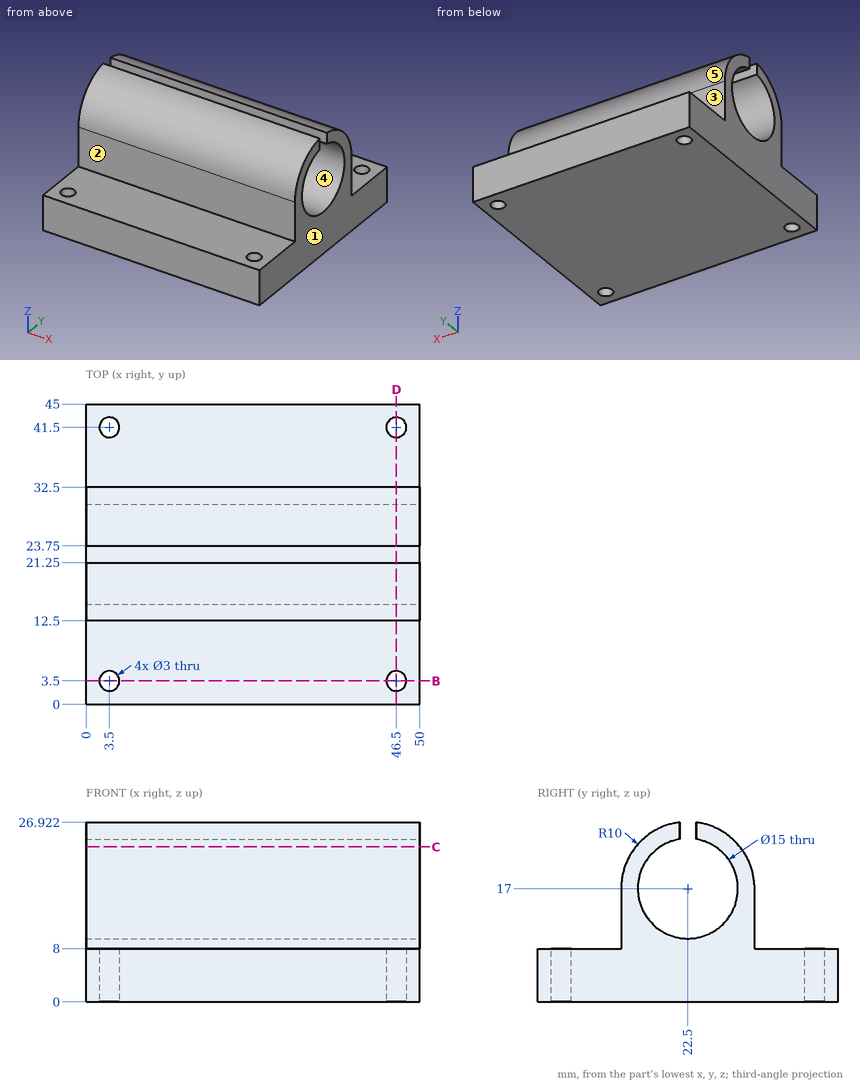
Can you work these out from the drawing? Everything is in mm from the part's minimum corner. A direction names the side the tool comes from. Round coordinates to 2 decimals unless told otherwise and drop trailing zeros. Write each loop counter-clockwise with the first axis right and the second up, starting at its lowest first coordinate (ties: lowest second). Pieces come first, ordered by that corner, then holes.
1. If we mould it in two halves opening along Z, with no side actions, what happens to the marked faces 3, 4 and 5? For each: released by +Z, released by -Z, zero draft, split by the parting line, or undercut.
2. For the marked faces 1 and 2, which set-ups out of +Z, -Z, +X, -X, +Y, -Y let a thin tool reach every point of the face, with its end or its side?
3. Will these pins go through, and if not, where does the flat tip stop? pin 1 Ø2.5 at (x, y) = (3.5, 3.5) entering from -Z; pin 2 Ø1.3 at (x, z) = (22, 25.5) entering from -Y (1 decimal); pin 3 Ø4 at (x, z) = (32, 13.5) entering from -Y; pin 4 Ø4 at (x, y) = (22.5, 7.5) entering from +Z.
4. Suppose I cut it at B-B (y = 3.5). List the corners of the cut face in (x, z) for me.
5. Suppose I cut it at D-D (x = 46.5). State how many separate pieces and enclosed holes the cut face has, and give its area (3 significant figures).
6. Suppose I cut it at C-C (z = 23.25). List the corners of the cut face in (x, y) for me (1 decimal), and give its area (3 significant figures).
7. I need wall thicknesses on L1, parallel to Y at x = 3.5, z = 3; L2, parallel to Y at x = 39, z = 17; L3, parallel to Y at x = 47, z = 1.75 (1 decimal). Which ranges of each line are inside material? Lowest first, please.
Answer sheet:
1. face 3: zero draft
1. face 4: undercut
1. face 5: released by +Z
2. face 1: +Z, -Z, +X, +Y, -Y
2. face 2: +Z, +X, -X, -Y
3. pin 1: passes through
3. pin 2: stops at y = 16.3
3. pin 3: stops at y = 12.5
3. pin 4: stops at z = 8
4. outline: (0, 0) - (2, 0) - (2, 8) - (0, 8) - close; (5, 0) - (45, 0) - (45, 8) - (5, 8) - close; (48, 0) - (50, 0) - (50, 8) - (48, 8) - close
5. separate pieces: 3
5. enclosed holes: 0
5. area: 466 mm2
6. outline: (0, 14.7) - (50, 14.7) - (50, 18.4) - (0, 18.4) - close; (0, 26.6) - (50, 26.6) - (50, 30.3) - (0, 30.3) - close
6. area: 366 mm2
7. L1: y = 0 to 2, 5 to 40, 43 to 45
7. L2: y = 12.5 to 15, 30 to 32.5
7. L3: y = 0 to 2.1, 4.9 to 40.1, 42.9 to 45
